```python
from build123d import *

# Parameters (mm, degrees)
MODEL_W                 = 3
MODEL_H                 = 3
SALIENTE_EXTRUIR1_DEPTH = 3


with BuildPart() as part:
    # Model → Saliente-Extruir1 (new body)
    with BuildSketch(Plane.XY):
        with BuildLine():
            Line((9.478716471, 295.822349433), (9.478716471, 269.422349433))
            ThreePointArc((9.478716471, 269.422349433), (9.566584436, 269.210217399), (9.778716471, 269.122349433))
            Line((9.778716471, 269.122349433), (12.378716471, 269.122349433))
            Line((12.378716471, 269.122349433), (12.378716471, 266.422349433))
            ThreePointArc((12.378716471, 266.422349433), (12.466584436, 266.210217399), (12.678716471, 266.122349433))
            Line((12.678716471, 266.122349433), (15.278716471, 266.122349433))
            ThreePointArc((15.278716471, 266.122349433), (15.490848505, 266.210217399), (15.578716471, 266.422349433))
            Line((15.578716471, 266.422349433), (15.578716471, 269.122349433))
            Line((15.578716471, 269.122349433), (16.978716471, 269.122349433))
            Line((16.978716471, 269.122349433), (16.978716471, 273.622349433))
            ThreePointArc((16.978716471, 273.622349433), (17.418056299, 274.683009605), (18.478716471, 275.122349433))
            Line((18.478716471, 275.122349433), (45.478716471, 275.122349433))
            ThreePointArc((45.478716471, 275.122349433), (46.539376642, 274.683009605), (46.978716471, 273.622349433))
            Line((46.978716471, 273.622349433), (46.978716471, 269.122349433))
            Line((46.978716471, 269.122349433), (48.378716471, 269.122349433))
            Line((48.378716471, 269.122349433), (48.378716471, 266.422349433))
            ThreePointArc((48.378716471, 266.422349433), (48.466584436, 266.210217399), (48.678716471, 266.122349433))
            Line((48.678716471, 266.122349433), (51.278716471, 266.122349433))
            ThreePointArc((51.278716471, 266.122349433), (51.490848505, 266.210217399), (51.578716471, 266.422349433))
            Line((51.578716471, 266.422349433), (51.578716471, 269.122349433))
            Line((51.578716471, 269.122349433), (54.178716471, 269.122349433))
            ThreePointArc((54.178716471, 269.122349433), (54.390848505, 269.210217399), (54.478716471, 269.422349433))
            Line((54.478716471, 269.422349433), (54.478716471, 295.822349433))
            ThreePointArc((54.478716471, 295.822349433), (54.390848505, 296.034481468), (54.178716471, 296.122349433))
            Line((54.178716471, 296.122349433), (51.578716471, 296.122349433))
            Line((51.578716471, 296.122349433), (51.578716471, 298.822349433))
            ThreePointArc((51.578716471, 298.822349433), (51.490848505, 299.034481468), (51.278716471, 299.122349433))
            Line((51.278716471, 299.122349433), (48.678716471, 299.122349433))
            ThreePointArc((48.678716471, 299.122349433), (48.466584436, 299.034481468), (48.378716471, 298.822349433))
            Line((48.378716471, 298.822349433), (48.378716471, 296.122349433))
            Line((48.378716471, 296.122349433), (42.578716471, 296.122349433))
            Line((42.578716471, 296.122349433), (42.578716471, 298.822349433))
            ThreePointArc((42.578716471, 298.822349433), (42.490848505, 299.034481468), (42.278716471, 299.122349433))
            Line((42.278716471, 299.122349433), (39.678716471, 299.122349433))
            ThreePointArc((39.678716471, 299.122349433), (39.466584436, 299.034481468), (39.378716471, 298.822349433))
            Line((39.378716471, 298.822349433), (39.378716471, 296.122349433))
            Line((39.378716471, 296.122349433), (33.578716471, 296.122349433))
            Line((33.578716471, 296.122349433), (33.578716471, 298.822349433))
            ThreePointArc((33.578716471, 298.822349433), (33.490848505, 299.034481468), (33.278716471, 299.122349433))
            Line((33.278716471, 299.122349433), (30.678716471, 299.122349433))
            ThreePointArc((30.678716471, 299.122349433), (30.466584436, 299.034481468), (30.378716471, 298.822349433))
            Line((30.378716471, 298.822349433), (30.378716471, 296.122349433))
            Line((30.378716471, 296.122349433), (24.578716471, 296.122349433))
            Line((24.578716471, 296.122349433), (24.578716471, 298.822349433))
            ThreePointArc((24.578716471, 298.822349433), (24.490848505, 299.034481468), (24.278716471, 299.122349433))
            Line((24.278716471, 299.122349433), (21.678716471, 299.122349433))
            ThreePointArc((21.678716471, 299.122349433), (21.466584436, 299.034481468), (21.378716471, 298.822349433))
            Line((21.378716471, 298.822349433), (21.378716471, 296.122349433))
            Line((21.378716471, 296.122349433), (15.578716471, 296.122349433))
            Line((15.578716471, 296.122349433), (15.578716471, 298.822349433))
            ThreePointArc((15.578716471, 298.822349433), (15.490848505, 299.034481468), (15.278716471, 299.122349433))
            Line((15.278716471, 299.122349433), (12.678716471, 299.122349433))
            ThreePointArc((12.678716471, 299.122349433), (12.466584436, 299.034481468), (12.378716471, 298.822349433))
            Line((12.378716471, 298.822349433), (12.378716471, 296.122349433))
            Line((12.378716471, 296.122349433), (9.778716471, 296.122349433))
            ThreePointArc((9.778716471, 296.122349433), (9.566584436, 296.034481468), (9.478716471, 295.822349433))
        make_face()
        with Locations((13.978716471, 291.622349433)):
            Rectangle(MODEL_W, MODEL_H, mode=Mode.SUBTRACT)
        with Locations((22.978716471, 291.622349433)):
            Rectangle(MODEL_W, MODEL_H, mode=Mode.SUBTRACT)
        with Locations((31.978716471, 291.622349433)):
            Rectangle(MODEL_W, MODEL_H, mode=Mode.SUBTRACT)
        with Locations((13.978716471, 273.622349433)):
            Rectangle(MODEL_W, MODEL_H, mode=Mode.SUBTRACT)
        with Locations((13.978716471, 282.622349433)):
            Rectangle(MODEL_W, MODEL_H, mode=Mode.SUBTRACT)
        with Locations((22.978716471, 282.622349433)):
            Rectangle(MODEL_W, MODEL_H, mode=Mode.SUBTRACT)
        with Locations((31.978716471, 282.622349433)):
            Rectangle(MODEL_W, MODEL_H, mode=Mode.SUBTRACT)
        with Locations((49.978716471, 291.622349433)):
            Rectangle(MODEL_W, MODEL_H, mode=Mode.SUBTRACT)
        with Locations((49.978716471, 273.622349433)):
            Rectangle(MODEL_W, MODEL_H, mode=Mode.SUBTRACT)
        with Locations((49.978716471, 282.622349433)):
            Rectangle(MODEL_W, MODEL_H, mode=Mode.SUBTRACT)
        with Locations((40.978716471, 291.622349433)):
            Rectangle(MODEL_W, MODEL_H, mode=Mode.SUBTRACT)
        with Locations((40.978716471, 282.622349433)):
            Rectangle(MODEL_W, MODEL_H, mode=Mode.SUBTRACT)
    extrude(amount=SALIENTE_EXTRUIR1_DEPTH)


solid = part.part
```
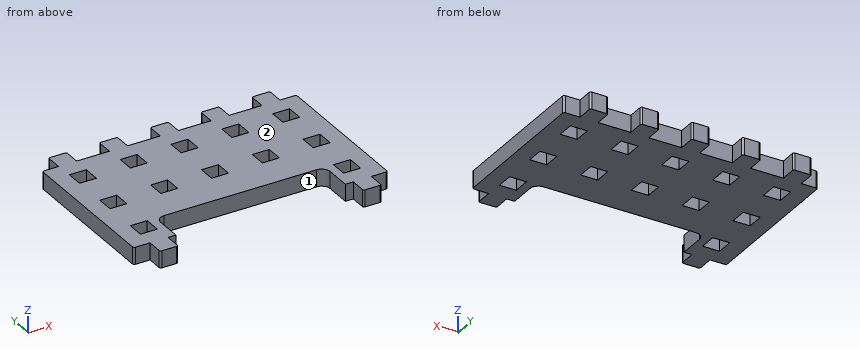
The listing builds one solid part. Answer for the finished solid, in the listing's coordinates (mm). Face numbers are marked on the shaded views. Coordinates: 2 decimals unless noted, no trailing zeros. Loops run counter-clockwise (first coordinate to the right, second up) from the corner with the lowest first, then second, coordinate; pieces in that order, holes last. Notation, with made-up numbers: (38, 5.25) - (81, 5.25) arc R17 ccw to (81, 35.25) - close; hole circle Ø3 at (1.5, 0). An arc over 180 degrees is marked (long way). Write item = value, one per line.
1) Determine the mould class of the marked faces 1 and 2 for opening direction X: pulls with the +X half, pulls with the -X half, needs draft (parallel to the pull), parting line crosses it, or undercut.
Responses:
face_1 = undercut
face_2 = needs draft
2) Section D-D (x = 32.5) is taken. Determine the outline of the cut face in (y, z), plus the area to 3 significant figures.
Responses:
outline = (275.12, 0) - (281.12, 0) - (281.12, 3) - (275.12, 3) - close; (284.12, 0) - (290.12, 0) - (290.12, 3) - (284.12, 3) - close; (293.12, 0) - (299.12, 0) - (299.12, 3) - (293.12, 3) - close
area = 54.0 mm^2
3) Find the intervals of material crossed by line 1 along Y through (x, z) = (31, 0.7); line 2 along X through (y, z) = (273, 2.55); line 3 along X through (y, z) = (297.5, 1.7), in increasing order.
Responses:
line_1 = 275.12 to 281.12, 284.12 to 290.12, 293.12 to 299.12
line_2 = 9.48 to 12.48, 15.48 to 16.98, 46.98 to 48.48, 51.48 to 54.48
line_3 = 12.38 to 15.58, 21.38 to 24.58, 30.38 to 33.58, 39.38 to 42.58, 48.38 to 51.58
4) Section C-C (y = 270.5) is taken. Determine the outline of the cut face in (x, z), plus the area to 3 significant figures.
Responses:
outline = (9.48, 0) - (16.98, 0) - (16.98, 3) - (9.48, 3) - close; (46.98, 0) - (54.48, 0) - (54.48, 3) - (46.98, 3) - close
area = 45.0 mm^2
5) Section A-A (y = 292) is taken. Determine the outline of the cut face in (x, z).
Responses:
outline = (9.48, 0) - (12.48, 0) - (12.48, 3) - (9.48, 3) - close; (15.48, 0) - (21.48, 0) - (21.48, 3) - (15.48, 3) - close; (24.48, 0) - (30.48, 0) - (30.48, 3) - (24.48, 3) - close; (33.48, 0) - (39.48, 0) - (39.48, 3) - (33.48, 3) - close; (42.48, 0) - (48.48, 0) - (48.48, 3) - (42.48, 3) - close; (51.48, 0) - (54.48, 0) - (54.48, 3) - (51.48, 3) - close
6) This flat-tipped pin is pushed along its axis until it touches: P1, Ø1.3, axis at y = 268, z = 2, coming from the -X side. Where does it stop, or does it pass through?
Responses:
P1 = 12.38
7) Section B-B (x = 14) is taken. Determine the outline of the cut face in (y, z).
Responses:
outline = (266.12, 0) - (272.12, 0) - (272.12, 3) - (266.12, 3) - close; (275.12, 0) - (281.12, 0) - (281.12, 3) - (275.12, 3) - close; (284.12, 0) - (290.12, 0) - (290.12, 3) - (284.12, 3) - close; (293.12, 0) - (299.12, 0) - (299.12, 3) - (293.12, 3) - close
